from build123d import *

# Parameters (mm, degrees)
SKETCH1_R           = 25.5
BOSS_EXTRUDE1_DEPTH = 35
SKETCH2_W           = 20.3
SKETCH2_H           = 20.3
CUT_EXTRUDE1_DEPTH  = 97.40539404
BOSS_EXTRUDE2_DEPTH = 70
SKETCH4_R           = 3.15
CUT_EXTRUDE2_DEPTH  = 20
SKETCH5_R           = 7
CUT_EXTRUDE3_DEPTH  = 8
FILLET1_R           = 1
FILLET2_R           = 10
CHAMFER1_SIZE       = 0.5


with BuildPart() as part:
    # Sketch1 → Boss-Extrude1 (new, symmetric)
    with BuildSketch(Plane(origin=(0, 0, 0), x_dir=(1, 0, 0), z_dir=(0, 1, 0))):
        with BuildLine():
            Line((-37, 0), (-37, -55))
            Line((-37, -55), (37, -55))
            Line((37, -55), (37, 0))
            ThreePointArc((37, 0), (0, 37), (-37, 0))
        make_face()
        with Locations(Location((0, 0, 0), (0, 0, 270))):
            Circle(SKETCH1_R, mode=Mode.SUBTRACT)
    extrude(amount=BOSS_EXTRUDE1_DEPTH, both=True)

    # Sketch2 → Cut-Extrude1 (cut, through all)
    with BuildSketch(Plane(origin=(0, 35, 0), x_dir=(1, 0, 0), z_dir=(0, 1, 0))):
        with Locations((-26.85, -44.85)):
            Rectangle(SKETCH2_W, SKETCH2_H)
        with Locations((26.85, -44.85)):
            Rectangle(SKETCH2_W, SKETCH2_H)
    extrude(amount=-CUT_EXTRUDE1_DEPTH, mode=Mode.SUBTRACT)

    # Sketch3 → Boss-Extrude2 (add)
    with BuildSketch(Plane(origin=(0, 35, 0), x_dir=(1, 0, 0), z_dir=(0, 1, 0))):
        Polygon((-37, -34.7), (-37, -55), (-49, -55), (-49, -22.7), (-37, -10.7), align=None)
    boss_extrude2 = extrude(amount=-BOSS_EXTRUDE2_DEPTH)

    # Sketch4 → Cut-Extrude2 (cut)
    with BuildSketch(Plane.ZY.offset(49)):
        with Locations((45, 22.5)):
            Circle(SKETCH4_R)
        with Locations((45, -22.5)):
            Circle(SKETCH4_R)
    cut_extrude2 = extrude(amount=-CUT_EXTRUDE2_DEPTH, mode=Mode.SUBTRACT)

    # Sketch5 → Cut-Extrude3 (cut)
    with BuildSketch(Plane.ZY.offset(49)):
        with Locations((45, 22.5)):
            Circle(SKETCH5_R)
        with Locations((45, -22.5)):
            Circle(SKETCH5_R)
    cut_extrude3 = extrude(amount=-CUT_EXTRUDE3_DEPTH, mode=Mode.SUBTRACT)

    # Mirror5: Boss-Extrude2, Cut-Extrude2, Cut-Extrude3 across plane
    add(boss_extrude2.mirror(Plane(origin=(0, 0, 0), x_dir=(0, 0, 1), z_dir=(1, 0, 0))))
    add(cut_extrude2.mirror(Plane(origin=(0, 0, 0), x_dir=(0, 0, 1), z_dir=(1, 0, 0))), mode=Mode.SUBTRACT)
    add(cut_extrude3.mirror(Plane(origin=(0, 0, 0), x_dir=(0, 0, 1), z_dir=(1, 0, 0))), mode=Mode.SUBTRACT)

    # Fillet1
    fillet1_edges = [part.edges().sort_by_distance(p)[0] for p in [
        (-37, 0, 34.7),
        (-16.7, 0, 34.7),
        (37, 0, 34.7),
        (16.7, 0, 34.7),
    ]]
    fillet(fillet1_edges, radius=FILLET1_R)

    # Fillet2
    fillet2_edges = [part.edges().sort_by_distance(p)[0] for p in [
        (-37, 0, 10.7),
        (-49, 0, 22.7),
        (49, 0, 22.7),
        (37, 0, 10.7),
    ]]
    fillet(fillet2_edges, radius=FILLET2_R)

    # Chamfer1
    chamfer1_edges = [part.edges().sort_by_distance(p)[0] for p in [
        (16.7, 35, 45.35),
        (16.7, -35, 45.35),
        (26.85, 35, 34.7),
        (26.85, -35, 34.7),
        (37, -35, 45.35),
        (-26.85, 35, 34.7),
        (-26.85, -35, 34.7),
        (0, -35, -25.5),
        (-37, -35, 45.35),
        (0, 35, -25.5),
        (16.992893219, 35, 34.992893219),
        (16.992893219, -35, 34.992893219),
        (36.707106781, 35, 34.992893219),
        (36.707106781, -35, 34.992893219),
        (-16.992893219, 35, 34.992893219),
        (-16.992893219, -35, 34.992893219),
        (-36.707106781, 35, 34.992893219),
        (-36.707106781, -35, 34.992893219),
        (49, 35, 40.921067812),
        (43, 35, 16.7),
        (37, 35, 3.278932188),
        (-43, 35, 16.7),
        (-49, 35, 40.921067812),
        (-48.238795325, 35, 23.0153013),
        (48.238795325, 35, 23.0153013),
        (43, -35, 16.7),
        (-43, -35, 16.7),
        (37, -35, 3.278932188),
        (-48.238795325, -35, 23.0153013),
        (48.238795325, -35, 23.0153013),
        (37.761204675, 35, 10.3846987),
        (37.761204675, -35, 10.3846987),
        (-37.761204675, 35, 10.3846987),
        (-37.761204675, -35, 10.3846987),
        (0, -35, 55),
        (0, 35, 55),
        (-16.7, -35, 45.35),
        (-16.7, 35, 45.35),
        (-37, 35, 45.35),
        (0, 35, -37),
        (-43, 35, 55),
        (-43, -35, 55),
        (-49, -35, 40.921067812),
        (-37, -35, 3.278932188),
        (0, -35, -37),
        (37, 35, 45.35),
        (43, -35, 55),
        (43, 35, 55),
        (49, -35, 40.921067812),
        (-37, 35, 3.278932188),
    ]]
    chamfer(chamfer1_edges, length=CHAMFER1_SIZE)


solid = part.part
Verification items for the finished model (mm, model axes). A direction names the side the tool comes from. Coordinates: 2 decimals unless noted, no trailing zeros. Order: outer loops, then holes, each group sorted by start corner. A loop starts at its lowest first (then second) coordinate and runs counter-clockwise, first axis right, second up. Notation, with made-up numbers: (27, 19) -> (47, 19) arc R26 cw to (47, 55) -> close; hole circle Ø3 at (33.25, 9.5). An arc over 180 degrees is marked (long way). Put each result on its own line as item: value. Start each with the question number.
1. Mould release check, pull along X, two halves, no side actions. Record for faces 4 (the flat face through (-27, 0, 34.7)), 5 (the conical face through (0.81, 34.86, -36.63)), 6 (the cylindrical face through (-45.06, 16.29, 48.23)): released by +X, released by -X, zero draft, split by the parting line, or undercut.
2. Material ranges on L1, parallel to X at y = -19.5, z = 38; L2, parallel to X at y = -27.5, z = 43; L3, parallel to Y at x = 43, z = 45, recorded low to high. Write a range as [from, to].
3. Go/stop test with flat-tipped pins: pin 1 Ø4 at (y, z) = (-22.5, 45) entering from +X; pin 2 Ø12.5 at (y, z) = (-22.5, 45) entering from +X; pin 3 Ø4 at (y, z) = (20, -22) entering from +X. Record where each tip stops, or that it passes through.
4. Cross-section at B-B, the plane x = 0. Record the boundary of the cut face in (y, z).
5. Cross-section at A-A, the plane y = -9.5. Record the boundary of the cut face in (x, z).
6. Access from +Z, -Z, +X, -X, +Y, -Y to the whole of each face (thin tool, end or side, straight path). Record for faces 1 (the cylindrical face through (-39.028, -24.417, 42.5)), 2 (the cylindrical face through (39.028, -24.417, 42.5)), 3 (the flat face through (-37, 0, 45)).
7. Cross-section at C-C, the plane z = 45. Count the separate pieces of the cut face and the enclosed holes in it, then the cut area to 3 significant figures.
Computed:
1. face 4: undercut
1. face 5: split by the parting line
1. face 6: zero draft
2. L1: [-49, -37], [-16.7, 16.7], [37, 49]
2. L2: [-41, -37], [-16.7, 16.7], [37, 41]
2. L3: [-35, -29.5], [-15.5, 15.5], [29.5, 35]
3. pin 1: x = 16.7
3. pin 2: x = 41
3. pin 3: x = 31.13
4. outline: (-35, -36.5) -> (-34.5, -37) -> (34.5, -37) -> (35, -36.5) -> (35, -26) -> (34.5, -25.5) -> (-34.5, -25.5) -> (-35, -26) -> close; (-35, 26) -> (-34.5, 25.5) -> (34.5, 25.5) -> (35, 26) -> (35, 54.5) -> (34.5, 55) -> (-34.5, 55) -> (-35, 54.5) -> close
5. outline: (-49, 26.84) arc R10 ccw to (-46.07, 19.77) -> (-39.93, 13.63) arc R10 cw to (-37, 6.56) -> (-37, 0) arc R37 ccw to (37, 0) -> (37, 6.56) arc R10 cw to (39.93, 13.63) -> (46.07, 19.77) arc R10 ccw to (49, 26.84) -> (49, 55) -> (37, 55) -> (37, 35.7) arc R1 cw to (36, 34.7) -> (17.7, 34.7) arc R1 cw to (16.7, 35.7) -> (16.7, 55) -> (-16.7, 55) -> (-16.7, 35.7) arc R1 cw to (-17.7, 34.7) -> (-36, 34.7) arc R1 cw to (-37, 35.7) -> (-37, 55) -> (-49, 55) -> close; hole circle Ø51 at (0, 0)
6. face 1: -X
6. face 2: +X
6. face 3: +Z, +Y, -Y
7. separate pieces: 7
7. enclosed holes: 0
7. area: 3,470 mm2
